Build history of the part. All positions in model axes, mm. Coordinates: 2 decimals unless noted, no trailing zeros. Loops run counter-clockwise (first coordinate to the right, second up) from the corner with the lowest first, then second, coordinate; pieces in that order, holes last.
Item 1: Drill centre lines: line 1 along Z through (x, y) = (0, -0.3); line 2 along Z through (x, y) = (-1.5, -0.65); line 3 along X through (y, z) = (-0.5, 55). Where is each one in solid material? Low to high.
Item 2: Mould opens along Z. For faces 1 (the face through (-0.187, -0.493, 63.918)), 2 (the face through (-0.54, -0.49, 57.86)), 3 (the face through (-0.54, -0.49, 2.44)), 4 (the face through (0, -1, 28)) say: released by +Z, released by -Z, zero draft, split by the parting line, or undercut.
Item 3: Cut at D-D (x = -3.5). List the corners of the cut face in (y, z), and give its area (3 significant figures).
Item 4: Flat gauge pin, fed straight in: pin 1 (5 mm diameter, centred on x = -4.5, z = 46.5, fed in from +Y). Where does the tip first touch, or does it go through?
Item 5: Cut at B-B (z = 1). List the corners of the cut face in (x, y).
Item 6: Cut at C-C (y = -0.8). List the corners of the cut face in (x, z).
Item 7: Cut at A-A (x = 0). List the corners of the cut face in (y, z).
Solid Edge part; units mm, degrees
sketch "Sketch1" plane through (0, 0, 0) normal (0, -1, 0) x (1, 0, 0)
  line L0 (8.5, 0) -> (8.5, 55.42)
  line L1 (-8.5, 55.42) -> (-8.5, 0)
  arc A0 (-8.5, 55.42) -> (8.5, 55.42) centre (0, 55.42) cw
  arc A1 (8.5, 0) -> (-8.5, 0) centre (0, 0) cw
  circle A2 centre (0, 55.42) radius 2.5
  circle A3 centre (0, 0) radius 2.5
extrude "Protrusion1" add sketch "Sketch1" along normal blind 1
Filled sheet:
1. line 1: z = -8.5 to -2.5, 2.5 to 52.92, 57.92 to 63.92
1. line 2: z = -8.37 to -2, 2 to 53.42, 57.42 to 63.79
1. line 3: x = -8.5 to -2.46, 2.46 to 8.5
2. face 1: released by +Z
2. face 2: undercut
2. face 3: undercut
2. face 4: zero draft
3. outline: (-1, -7.75) - (0, -7.75) - (0, 63.17) - (-1, 63.17) - close
3. area: 70.9 mm2
4. pin 1: stops at y = 0
5. outline: (-8.5, -1) - (-2.29, -1) - (-2.29, 0) - (-8.5, 0) - close; (2.29, -1) - (8.5, -1) - (8.5, 0) - (2.29, 0) - close
6. outline: (-8.5, 0) arc R8.5 ccw to (8.5, 0) - (8.5, 55.42) arc R8.5 ccw to (-8.5, 55.42) - close; hole circle Ø5 at (0, 0); hole circle Ø5 at (0, 55.42)
7. outline: (-1, -8.5) - (0, -8.5) - (0, -2.5) - (-1, -2.5) - close; (-1, 2.5) - (0, 2.5) - (0, 52.92) - (-1, 52.92) - close; (-1, 57.92) - (0, 57.92) - (0, 63.92) - (-1, 63.92) - close
